Here's how the part is built. I have some questions about the finished solid (model axes, mm). Round coordinates to 2 decimals unless told otherwise and drop trailing zeros. Write each loop counter-clockwise with the first axis right and the second up, starting at its lowest first coordinate (ties: lowest second). Pieces come first, ordered by that corner, then holes. Notation, with made-up numbers: (-14.5, 4) -> (22.5, 4) arc R31 cw to (22.5, 40) -> close; hole circle Ø10 at (19, -16.75). An arc over 180 degrees is marked (long way). Answer in a Markdown table with one row per item.
from build123d import *

# Parameters (mm, degrees)
SKETCH1_R           = 1
BOSS_EXTRUDE1_DEPTH = 8


with BuildPart() as part:
    # Sketch1 → Boss-Extrude1 (new body)
    with BuildSketch(Plane(origin=(0, 0, 0), x_dir=(1, 0, 0), z_dir=(0, 1, 0))):
        with BuildLine():
            Line((-62.675339064, 42.746325997), (77.324660936, 42.746325997))
            Line((77.324660936, 42.746325997), (77.324660936, -25.253674003))
            Line((77.324660936, -25.253674003), (9.324660936, -25.253674003))
            ThreePointArc((9.324660936, -25.253674003), (-6.675339064, -9.253674003), (-22.675339064, -25.253674003))
            Line((-22.675339064, -25.253674003), (-62.675339064, -25.253674003))
            Line((-62.675339064, -25.253674003), (-62.675339064, 42.746325997))
        make_face()
        with Locations((-32.675339064, 32.746325997)):
            Circle(SKETCH1_R, mode=Mode.SUBTRACT)
        with Locations((-32.675339064, -15.253674003)):
            Circle(SKETCH1_R, mode=Mode.SUBTRACT)
        with Locations((52.324660936, 32.746325997)):
            Circle(SKETCH1_R, mode=Mode.SUBTRACT)
        with Locations((52.324660936, -15.253674003)):
            Circle(SKETCH1_R, mode=Mode.SUBTRACT)
    extrude(amount=BOSS_EXTRUDE1_DEPTH)


solid = part.part
1) I need wall thicknesses on line 1 (X direction, y = 7.25, z = 22); line 2 (Z direction, x = 4.5, y = 1.75). Which ranges of each line are inside material? Lowest first, please. Write a range as [from, to].
Response:
| item | result |
|---|---|
| line 1 | x = [-62.68, -22.34], [8.99, 77.32] |
| line 2 | z = [-42.75, 13.8] |
2) I want a section at B-B, the plane x = -3. List the corners of the cut face in (y, z) for me, and give its area (3 significant figures).
Response:
| item | result |
|---|---|
| outline | (0, -42.75) -> (8, -42.75) -> (8, 9.68) -> (0, 9.68) -> close |
| area | 419 mm^2 |
3) For pin 1 (1.2 mm diameter, centred on x = 52.32, z = 15.25, fed in from -Y), with a flat end and sliding along its axis, tell me the tip position at first contact or that it passes through.
Response:
| item | result |
|---|---|
| pin 1 | passes through |
4) I want a section at A-A, the plane y = 4. List the corners of the cut face in (x, z) for me, and give its area (3 significant figures).
Response:
| item | result |
|---|---|
| outline | (-62.68, -42.75) -> (77.32, -42.75) -> (77.32, 25.25) -> (9.32, 25.25) arc R16 cw to (-22.68, 25.25) -> (-62.68, 25.25) -> close; hole circle Ø2 at (-32.68, -32.75); hole circle Ø2 at (-32.68, 15.25); hole circle Ø2 at (52.32, -32.75); hole circle Ø2 at (52.32, 15.25) |
| area | 9,110 mm^2 |
